Autodesk Inventor part; units mm, degrees
ref_plane "YZ Plane" through (0, 0, 0) normal (1, 0, 0) x (0, 1, 0)
ref_plane "XZ Plane" through (0, 0, 0) normal (0, 1, 0) x (-1, 0, 0)
ref_plane "XY Plane" through (0, 0, 0) normal (0, 0, 1) x (1, 0, 0)
sketch "Sketch1" plane through (0, 0, 0) normal (0, 0, 1) x (1, 0, 0)
  line L0 (0, 0) -> (127, 0)
  line L1 (127, 0) -> (127, 31.75)
  line L2 (127, 31.75) -> (0, 31.75)
  line L3 (0, 31.75) -> (0, 0)
  circle A0 centre (114.3, 15.875) radius 3.3655
  circle A1 centre (63.5, 15.875) radius 3.3655
  circle A2 centre (12.7, 15.875) radius 3.3655
  dimension "d0" = 127
  dimension "d1" = 31.75
  dimension "d2" = 6.731
  dimension "d3" = 12.7
  dimension "d4" = 15.875
  dimension "d7" = 50.8
extrude "Plate1" add sketch "Sketch1" along normal blind 3.048
fillet "Corner Round1" radius 6.35 4 edges at (0, 31.75, 1.524) (0, 0, 1.524) (127, 31.75, 1.524) (127, 0, 1.524)
equation "\"d4\" = 0.5 * d1"
equation "\"BendRadius\" = Thickness"
equation "\"BendReliefWidth\" = Thickness"
equation "\"BendReliefDepth\" = 0.5 * Thickness"
equation "\"CornerReliefSize\" = 4 * Thickness"
equation "\"MinimumRemnant\" = 2 * Thickness"
equation "\"TransitionRadius\" = BendRadius"
equation "\"JacobiRadiusSize\" = BendRadius"
equation "\"GapSize\" = Thickness"
equation "\"d12\" = BendRadius"
properties part number "Super1"
For this review, take the finished solid that the model builds, in its own axes (mm). Coordinates: 2 decimals unless noted, no trailing zeros. Write each loop counter-clockwise with the first axis right and the second up, starting at its lowest first coordinate (ties: lowest second). Pieces come first, ordered by that corner, then holes. Notation, with made-up numbers: (-36.5, 15.5) -> (-24.5, 15.5) arc R33 cw to (-24.5, 45.5) -> close; hole circle Ø8 at (87.25, -20.75). An arc over 180 degrees is marked (long way). Put each result on its own line as item: value.
Q1. Take a section at B-B, the plane z = 1.8. Count the separate pieces of the cut face and the enclosed holes in it, then the cut area to 3 significant figures.
From the geometry:
separate pieces: 1
enclosed holes: 3
area: 3,890 mm2
Q2. Wall thickness on L1, parallel to Y at x = 114.3, z = 1.65; L2, parallel to X at y = 14.5, z = 1.35; L3, parallel to X at y = 13.5, z = 2.7: over which ranges is each line inside the solid? List them lowest first.
From the geometry:
L1: y = 0 to 12.51, 19.24 to 31.75
L2: x = 0 to 9.63, 15.77 to 60.43, 66.57 to 111.23, 117.37 to 127
L3: x = 0 to 10.32, 15.08 to 61.12, 65.88 to 111.92, 116.68 to 127
Q3. The part is to be moulded in two halves that separate along Y. For faces 1 (the cylindrical face through (117.51, 14.86, 1.5)), 2 (the cylindrical face through (125.09, 1.81, 1.55)), 3 (the flat face through (0, 16, 2)), say which applies: +Y half, -Y half, draft (parallel to the pull), parting line (faces both ways), or undercut.
From the geometry:
face 1: undercut
face 2: -Y half
face 3: draft
Q4. Take a section at C-C, the plane y = 2. State the section outline as (x, z) points, then the cut area to 3 significant figures.
From the geometry:
outline: (1.72, 0) -> (125.28, 0) -> (125.28, 3.05) -> (1.72, 3.05) -> close
area: 377 mm2
Q5. Take a section at A-A, the plane x = 63.5. State the section outline as (y, z) points, then the cut area to 3 significant figures.
From the geometry:
outline: (0, 0) -> (12.51, 0) -> (12.51, 3.05) -> (0, 3.05) -> close; (19.24, 0) -> (31.75, 0) -> (31.75, 3.05) -> (19.24, 3.05) -> close
area: 76.3 mm2
